Could you check a few things on this drawing? It's one solid part, dimensions in mm from its lowest x, y, z. A direction names the side the tool comes from. Give positions to 0.01 mm unless a question says otherwise; leave off trailing zeros.
Q1. I'm going to push flat-ended pins straight in: P1, Ø2, axis at x = 22, z = 4, coming from the -Y side (1 decimal); P2, Ø3, axis at y = 8, z = 4, coming from the +X side; P3, Ø3, axis at x = 28, z = 6.5, coming from the -Y side. Where does each tip first touch, or does it pass through?
Q2. Thinking about a two-plate mould opening in Y: for the marked faces 3, 4, 5 and 6, which applies, pulls with the +Y half, pulls with the -Y half, needs draft (parallel to the pull), parting line crosses it, or undercut?
Q3. I need wall thicknesses on probe 1 along Y at (x, z) = (15.5, 7.25) (1 decimal); probe 2 along X at (y, z) = (19, 2.75) (1 decimal); probe 3 along X at (y, z) = (21.5, 7.5). Which ranges of each line are inside material? Lowest first, please.
Q4. For the marked faces 1 and 2, which set-ups out of +Z, -Z, +X, -X, +Y, -Y let a thin tool reach every point of the face, with its end or its side?
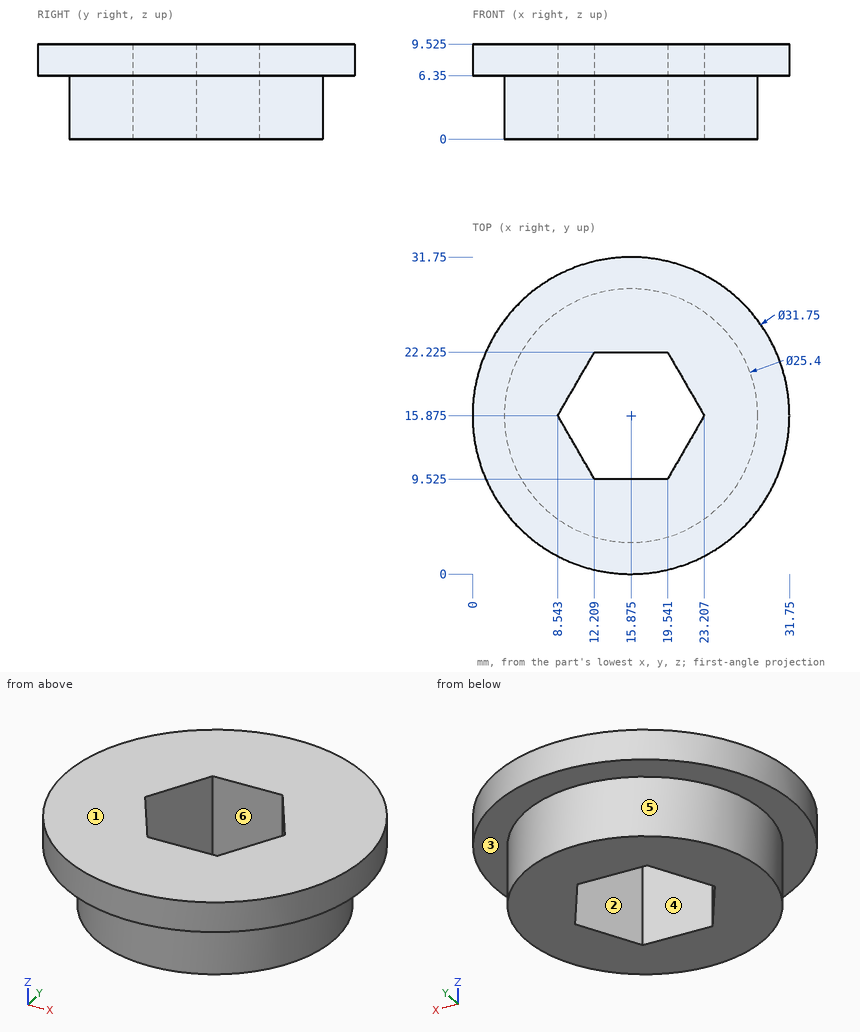
Solutions:
1. P1: stops at y = 4.3
1. P2: stops at x = 26.86
1. P3: stops at y = 4.08
2. face 3: needs draft
2. face 4: undercut
2. face 5: parting line crosses it
2. face 6: undercut
3. probe 1: y = 0 to 9.5, 22.2 to 31.7
3. probe 2: x = 3.6 to 10.3, 21.4 to 28.2
3. probe 3: x = 1.03 to 11.79, 19.96 to 30.72
4. face 1: +Z, +X, -X, +Y, -Y
4. face 2: +Z, -Z
